Geometry check sheet. Reference: the model listing, model coordinates, mm. Face numbers are marked on the shaded views. A direction names the side the tool comes from. Coordinates: 2 decimals unless noted, no trailing zeros. Loops run counter-clockwise (first coordinate to the right, second up) from the corner with the lowest first, then second, coordinate; pieces in that order, holes last.
from build123d import *
from OCP.BRepFilletAPI import BRepFilletAPI_MakeChamfer

# Parameters (mm, degrees)
EXTRUDE_1_DEPTH                  = 11.1
CUT_EXTRUDE_1_DEPTH              = 7.7
SKETCH_13_R                      = 2.175
CUT_EXTRUDE_9_DEPTH              = 7.7
CUT_EXTRUDE_10_REACH             = 14.986
SKETCH_3_W                       = 1.5
SKETCH_3_H                       = 1.2
CUT_EXTRUDE_10_DIRECTION_2_REACH = 14.986
SKETCH_14_W                      = 1.5
SKETCH_14_H                      = 4
EXTRUDE_5_DEPTH                  = 1.2
EXTRUDE_START                    = 6.5
SKETCH_5_R                       = 2.175
EXTRUDE_3_DEPTH                  = 6.5
SKETCH_10_R                      = 2.15
CUT_EXTRUDE_7_DEPTH              = 6.5
SKETCH_16_R                      = 1.25
SKETCH_18_R                      = 1.25
EXTRUDE_7_DEPTH                  = 2
EXTRUDE_8_DEPTH                  = 8.1
EXTRUDE_START_2                  = -2.1
EXTRUDE_9_DEPTH                  = 2.1
SKETCH_21_W                      = 10.2
SKETCH_21_H                      = 2.025
EXTRUDE_12_DEPTH                 = 1
SKETCH_22_W                      = 0.6
SKETCH_22_H                      = 1.6
CUT_EXTRUDE_12_DEPTH             = 21.530769591
SKETCH_23_W                      = 0.7
SKETCH_23_H                      = 0.7
CUT_EXTRUDE_13_DEPTH             = 21.530769591
EXTRUDE_13_DEPTH                 = 2
EXTRUDE_13_DEPTH_BACK            = 7.6
SKETCH_24_W                      = 0.6
SKETCH_24_H                      = 1.6
EXTRUDE_14_DEPTH                 = 0.5
CHAMFER_2_SIZE                   = 1
CHAMFER_2_SIZE2                  = 0.577350269
CHAMFER_3_SIZE                   = 0.5
SKETCH_26_W                      = 9.9
SKETCH_26_H                      = 1.6
CUT_EXTRUDE_14_DEPTH             = 0.7
FILLET_4_R                       = 0.3
CUT_EXTRUDE_15_DEPTH             = 20.811738944
CUT_EXTRUDE_15_DEPTH_BACK        = 20.811738944
FILLET_5_R                       = 1


with BuildPart() as part:
    # Эскиз1 → Бобышка-Вытянуть1 (new body)
    with BuildSketch(Plane.XY):
        Polygon((-7.75, 1.221572875), (-7.75, -1.221572875), (-4.921572875, -4.05), (7.75, -4.05), (7.75, 4.05), (-4.921572875, 4.05), align=None)
    extrude(amount=EXTRUDE_1_DEPTH)

    # Эскиз2 → Вырез-Вытянуть1 (cut)
    with BuildSketch(Plane(origin=(0, 0, 0), x_dir=(-1, 0, 0), z_dir=(0, 0, -1))):
        Polygon((-7.75, 4.05), (-7.75, -4.05), (4.921572875, -4.05), (7.75, -1.221572875), (7.75, 1.221572875), (4.921572875, 4.05), align=None)
        Polygon((4.631623382, 3.35), (7.05, 0.931623382), (7.05, -0.931623382), (4.631623382, -3.35), (-7.05, -3.35), (-7.05, 3.35), align=None, mode=Mode.SUBTRACT)
    extrude(amount=-CUT_EXTRUDE_1_DEPTH, mode=Mode.SUBTRACT)

    # Эскиз13 → Вырез-Вытянуть9 (cut)
    with BuildSketch(Plane(origin=(0, 0, 0), x_dir=(-1, 0, 0), z_dir=(0, 0, -1))):
        with Locations((-3.6, 0)):
            Circle(SKETCH_13_R)
        with Locations((3.6, 0)):
            Circle(SKETCH_13_R)
    extrude(amount=-CUT_EXTRUDE_9_DEPTH, mode=Mode.SUBTRACT)

    # Вырез-Вытянуть10: up to this face of the body (flat: up to its plane)
    cut_extrude_10_end = Plane(part.part.faces().sort_by_distance((-3.6, 0, 7.7))[0])
    # Эскиз3 → Вырез-Вытянуть10 (cut, up to the picked face)
    with BuildSketch(Plane(origin=(0, 0, 1.5), x_dir=(-1, 0, 0), z_dir=(0, 0, -1)), mode=Mode.PRIVATE) as cut_extrude_10_sk1:
        with Locations((0, 2.75)):
            Rectangle(SKETCH_3_W, SKETCH_3_H)
    cut_extrude_10_tool1 = split(extrude(cut_extrude_10_sk1.sketch, amount=-CUT_EXTRUDE_10_REACH, mode=Mode.PRIVATE), bisect_by=cut_extrude_10_end, keep=Keep.BOTH, mode=Mode.PRIVATE)
    add(cut_extrude_10_tool1.solids().sort_by(Axis((0, 2.75, 1.5), (0, 0, 1)))[0], mode=Mode.SUBTRACT)

    # Вырез-Вытянуть10 direction 2: up to this face of the body (flat: up to its plane)
    cut_extrude_10_direction_2_end = Plane(part.part.faces().sort_by_distance((0.620013342, 0, 0))[0])
    # Эскиз3 → Вырез-Вытянуть10 direction 2 (cut, up to the picked face)
    with BuildSketch(Plane(origin=(0, 0, 1.5), x_dir=(-1, 0, 0), z_dir=(0, 0, -1)), mode=Mode.PRIVATE) as cut_extrude_10_direction_2_sk1:
        with Locations((0, 2.75)):
            Rectangle(SKETCH_3_W, SKETCH_3_H)
    cut_extrude_10_direction_2_tool1 = split(extrude(cut_extrude_10_direction_2_sk1.sketch, amount=CUT_EXTRUDE_10_DIRECTION_2_REACH, mode=Mode.PRIVATE), bisect_by=cut_extrude_10_direction_2_end, keep=Keep.BOTH, mode=Mode.PRIVATE)
    add(cut_extrude_10_direction_2_tool1.solids().sort_by(Axis((0, 2.75, 1.5), (0, 0, -1)))[0], mode=Mode.SUBTRACT)

    # Эскиз14 → Бобышка-Вытянуть5 (add)
    with BuildSketch(Plane(origin=(0, 0, 0), x_dir=(-1, 0, 0), z_dir=(0, 0, -1))):
        with Locations((0, 0.15)):
            Rectangle(SKETCH_14_W, SKETCH_14_H)
    extrude(amount=EXTRUDE_5_DEPTH)

    # Эскиз5 → Бобышка-Вытянуть3 (add)
    with BuildSketch(Plane(origin=(0, 0, 7.7), x_dir=(-1, 0, 0), z_dir=(0, 0, -1)).offset(EXTRUDE_START)):
        with Locations((3.6, 0)):
            Circle(SKETCH_5_R)
        with Locations((-3.6, 0)):
            Circle(SKETCH_5_R)
    extrude(amount=-EXTRUDE_3_DEPTH)

    # Эскиз10 → Вырез-Вытянуть7 (cut)
    with BuildSketch(Plane(origin=(0, 0, 1.2), x_dir=(-1, 0, 0), z_dir=(0, 0, -1))):
        with Locations((-3.6, 0)):
            Circle(SKETCH_10_R)
        with Locations((3.6, 0)):
            Circle(SKETCH_10_R)
    extrude(amount=-CUT_EXTRUDE_7_DEPTH, mode=Mode.SUBTRACT)

    # По траектории1: sweep along a path in Эскиз17
    with BuildLine(Plane(origin=(0, 0, 0), x_dir=(0, 0, -1), z_dir=(1, 0, 0))) as sweep_1_path:
        ThreePointArc((-15.15, 4.05), (-13.963782464, 1.186217536), (-11.1, 0))
    # Эскиз16 → По траектории1 (sweep)
    with BuildSketch(Plane.XY.offset(11.1)):
        with Locations((3.6, 0)):
            Circle(SKETCH_16_R)
        with Locations((-3.6, 0)):
            Circle(SKETCH_16_R)
    sweep(path=sweep_1_path.line)

    # Эскиз18 → Бобышка-Вытянуть7 (add)
    with BuildSketch(Plane(origin=(0, 4.05, 0), x_dir=(1, 0, 0), z_dir=(0, 1, 0))):
        with Locations(Location((3.6, -15.15, 0), (0, 0, 270))):
            Circle(SKETCH_18_R)
        with Locations(Location((-3.6, -15.15, 0), (0, 0, 270))):
            Circle(SKETCH_18_R)
    extrude(amount=EXTRUDE_7_DEPTH)

    # Эскиз19 → Бобышка-Вытянуть8 (add)
    with BuildSketch(Plane(origin=(0, 4.05, 0), x_dir=(1, 0, 0), z_dir=(0, 1, 0))):
        with BuildLine():
            ThreePointArc((5.25, -17.2), (7.100752265, -14.396209945), (7.75, -11.1))
            Line((7.75, -11.1), (5.1, -11.1))
            Line((5.1, -11.1), (5.1, -15.15))
            ThreePointArc((5.1, -15.15), (3.6, -16.65), (2.1, -15.15))
            Line((2.1, -15.15), (2.1, -11.1))
            Line((2.1, -11.1), (-2.1, -11.1))
            Line((-2.1, -11.1), (-2.1, -15.15))
            ThreePointArc((-2.1, -15.15), (-3.6, -16.65), (-5.1, -15.15))
            Line((-5.1, -15.15), (-5.1, -11.1))
            Line((-5.1, -11.1), (-4.921572875, -11.1))
            Line((-4.921572875, -11.1), (-4.921572875, -7.7))
            Line((-4.921572875, -7.7), (-7.75, -7.7))
            Line((-7.75, -7.7), (-7.75, -11.1))
            ThreePointArc((-7.75, -11.1), (-7.100752265, -14.396209945), (-5.25, -17.2))
            Line((-5.25, -17.2), (5.25, -17.2))
        make_face()
    extrude(amount=-EXTRUDE_8_DEPTH)

    # Эскиз20 → Бобышка-Вытянуть9 (add)
    with BuildSketch(Plane.XZ.offset(4.05).offset(EXTRUDE_START_2)):
        with BuildLine():
            Line((-7.75, 7.7), (7.75, 7.7))
            Line((7.75, 7.7), (7.75, 11.1))
            ThreePointArc((7.75, 11.1), (7.100752265, 14.396209945), (5.25, 17.2))
            Line((5.25, 17.2), (-5.25, 17.2))
            ThreePointArc((-5.25, 17.2), (-7.100752265, 14.396209945), (-7.75, 11.1))
            Line((-7.75, 11.1), (-7.75, 7.7))
        make_face()
    extrude(amount=EXTRUDE_9_DEPTH)

    # Эскиз21 → Бобышка-Вытянуть12 (add)
    with BuildSketch(Plane(origin=(0, 4.05, 0), x_dir=(1, 0, 0), z_dir=(0, 1, 0))):
        with Locations((0, -12.1125)):
            Rectangle(SKETCH_21_W, SKETCH_21_H)
    extrude(amount=-EXTRUDE_12_DEPTH)

    # Эскиз22 → Вырез-Вытянуть12 (cut, through all)
    with BuildSketch(Plane(origin=(0, 4.05, 0), x_dir=(1, 0, 0), z_dir=(0, 1, 0))):
        with Locations((-6.75, -9.15)):
            Rectangle(SKETCH_22_W, SKETCH_22_H)
        with Locations((6.75, -9.15)):
            Rectangle(SKETCH_22_W, SKETCH_22_H)
    extrude(amount=-CUT_EXTRUDE_12_DEPTH, mode=Mode.SUBTRACT)

    # Эскиз23 → Вырез-Вытянуть13 (cut, through all)
    with BuildSketch(Plane(origin=(0, 4.05, 0), x_dir=(1, 0, 0), z_dir=(0, 1, 0))):
        with Locations((-7.4, -9.15)):
            Rectangle(SKETCH_23_W, SKETCH_23_H)
        with Locations((7.4, -9.15)):
            Rectangle(SKETCH_23_W, SKETCH_23_H)
    extrude(amount=-CUT_EXTRUDE_13_DEPTH, mode=Mode.SUBTRACT)

    # Эскиз24 → Бобышка-Вытянуть13 (add, two sides: drawn at the far end of the back side and taken through both)
    with BuildSketch(Plane(origin=(0, 4.05, 0), x_dir=(1, 0, 0), z_dir=(0, 1, 0)).offset(-EXTRUDE_13_DEPTH_BACK)):
        with Locations((-6.75, -9.15)):
            Rectangle(SKETCH_24_W, SKETCH_24_H)
        with Locations((6.75, -9.15)):
            Rectangle(SKETCH_24_W, SKETCH_24_H)
    extrude(amount=EXTRUDE_13_DEPTH + EXTRUDE_13_DEPTH_BACK)

    # Эскиз25 → Бобышка-Вытянуть14 (add)
    with BuildSketch(Plane(origin=(0, 4.05, 0), x_dir=(1, 0, 0), z_dir=(0, 1, 0))):
        Polygon((-6.15, -8.05), (-7.35, -8.05), (-7.35, -8.8), (-7.05, -8.8), (-7.05, -8.35), (-6.45, -8.35), (-6.45, -9.95), (-7.05, -9.95), (-7.05, -9.5), (-7.35, -9.5), (-7.35, -10.25), (-6.15, -10.25), align=None)
        Polygon((7.35, -8.05), (6.15, -8.05), (6.15, -10.25), (7.35, -10.25), (7.35, -9.5), (7.05, -9.5), (7.05, -9.95), (6.45, -9.95), (6.45, -8.35), (7.05, -8.35), (7.05, -8.8), (7.35, -8.8), align=None)
    extrude(amount=EXTRUDE_14_DEPTH)

    # Фаска2: one chamfer whose edges measure the first distance from different faces: ONE call of the kernel's chamfer builder (chamfer() names one face for all edges)
    chamfer_2_edges_1 = [part.edges().sort_by_distance(p)[0] for p in [
        (-6.75, 6.05, 9.95),
    ]]
    chamfer_2_side_1 = [part.faces().sort_by_distance(p)[0] for p in [
        (-6.75, 5.3, 9.95),
    ]]
    chamfer_2_edges_2 = [part.edges().sort_by_distance(p)[0] for p in [
        (-6.75, 6.05, 8.35),
    ]]
    chamfer_2_side_2 = [part.faces().sort_by_distance(p)[0] for p in [
        (-6.75, 5.3, 8.35),
    ]]
    chamfer_2_edges_3 = [part.edges().sort_by_distance(p)[0] for p in [
        (6.75, 6.05, 9.95),
    ]]
    chamfer_2_side_3 = [part.faces().sort_by_distance(p)[0] for p in [
        (6.75, 5.3, 9.95),
    ]]
    chamfer_2_edges_4 = [part.edges().sort_by_distance(p)[0] for p in [
        (6.75, 6.05, 8.35),
    ]]
    chamfer_2_side_4 = [part.faces().sort_by_distance(p)[0] for p in [
        (6.75, 5.3, 8.35),
    ]]
    chamfer_2 = BRepFilletAPI_MakeChamfer(part.part.solid().wrapped)
    for e in chamfer_2_edges_1:
        chamfer_2.Add(CHAMFER_2_SIZE, CHAMFER_2_SIZE2, e.wrapped, chamfer_2_side_1[0].wrapped)  # the first distance lies on this face
    for e in chamfer_2_edges_2:
        chamfer_2.Add(CHAMFER_2_SIZE, CHAMFER_2_SIZE2, e.wrapped, chamfer_2_side_2[0].wrapped)  # the first distance lies on this face
    for e in chamfer_2_edges_3:
        chamfer_2.Add(CHAMFER_2_SIZE, CHAMFER_2_SIZE2, e.wrapped, chamfer_2_side_3[0].wrapped)  # the first distance lies on this face
    for e in chamfer_2_edges_4:
        chamfer_2.Add(CHAMFER_2_SIZE, CHAMFER_2_SIZE2, e.wrapped, chamfer_2_side_4[0].wrapped)  # the first distance lies on this face
    add(Compound.cast(chamfer_2.Shape()), mode=Mode.REPLACE)

    # Фаска3
    chamfer_3_edges = [part.edges().sort_by_distance(p)[0] for p in [
        (3.6, 6.05, 13.9),
        (-3.6, 6.05, 13.9),
    ]]
    chamfer(chamfer_3_edges, length=CHAMFER_3_SIZE)

    # Эскиз26 → Вырез-Вытянуть14 (cut)
    with BuildSketch(Plane.XZ.offset(4.05)):
        with Locations((0, 9.15)):
            Rectangle(SKETCH_26_W, SKETCH_26_H)
    extrude(amount=-CUT_EXTRUDE_14_DEPTH, mode=Mode.SUBTRACT)

    # Скругление4
    fillet_4_edges = [part.edges().sort_by_distance(p)[0] for p in [
        (7.75, -4.05, 8.25),
        (-7.75, -4.05, 8.25),
        (7.05, 3.35, 3.85),
        (7.05, -3.35, 3.85),
        (-4.631623382, -3.35, 3.85),
        (-7.05, -0.931623382, 3.85),
        (-7.05, 0.931623382, 3.85),
        (-4.631623382, 3.35, 3.85),
        (4.95, -3.7, 9.95),
        (4.95, -3.7, 8.35),
        (-4.95, -3.7, 8.35),
        (-4.95, -3.7, 9.95),
    ]]
    fillet(fillet_4_edges, radius=FILLET_4_R)

    # Эскиз27 → Вырез-Вытянуть15 (cut, two sides: drawn at the far end of the back side and taken through both)
    with BuildSketch(Plane(origin=(0, 0, 0), x_dir=(0, 0, -1), z_dir=(1, 0, 0)).offset(-CUT_EXTRUDE_15_DEPTH_BACK)):
        with BuildLine():
            Line((-11.1, -4.05), (-17.2, -4.05))
            Line((-17.2, -4.05), (-17.2, -1.55))
            ThreePointArc((-17.2, -1.55), (-14.396209945, -3.400752265), (-11.1, -4.05))
        make_face()
    extrude(amount=CUT_EXTRUDE_15_DEPTH + CUT_EXTRUDE_15_DEPTH_BACK, mode=Mode.SUBTRACT)

    # Скругление5
    fillet_5_edges = [part.edges().sort_by_distance(p)[0] for p in [
        (7.75, -4.05, 10.3),
        (-7.75, -4.05, 10.3),
        (5.25, 1.25, 17.2),
        (-5.25, 1.25, 17.2),
        (7.027776856, -3.327776856, 14.568936562),
        (-7.027776856, -3.327776856, 14.568936562),
        (0, -1.55, 17.2),
    ]]
    fillet(fillet_5_edges, radius=FILLET_5_R)


solid = part.part
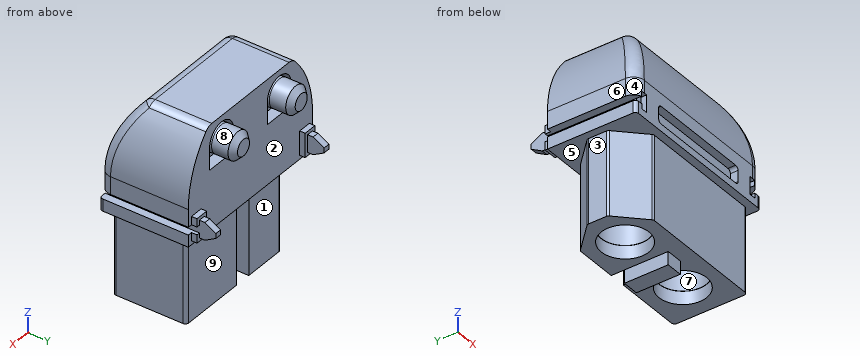
1) Depth check by flat-ended pin: pin 1 (0.9 mm diameter, centred on x = 3.5, z = 12.5, fed in from +Y); pin 2 (2 mm diameter, centred on y = 1, z = 7, fed in from +X); pin 3 (6 mm diameter, centred on x = 0, z = 14, fed in from +Y); pin 4 (0.6 mm diameter, centred on y = 0.5, z = -0.5, fed in from +X). Enter the tip coordinate at first touch or a pass-through.
Data:
pin 1: stops at y = 4.05
pin 2: stops at x = 7.75
pin 3: stops at y = 6.02
pin 4: stops at x = 0.75
2) Section check A-A on z = 4.5. Record the cut outline in (x, y), and give its area (3 significant figures).
Data:
outline: (-7.05, -0.81) arc R0.3 ccw to (-6.96, -1.02) - (-4.72, -3.26) arc R0.3 ccw to (-4.51, -3.35) - (6.75, -3.35) arc R0.3 ccw to (7.05, -3.05) - (7.05, 3.05) arc R0.3 ccw to (6.75, 3.35) - (0.75, 3.35) - (0.75, 2.15) - (-0.75, 2.15) - (-0.75, 3.35) - (-4.51, 3.35) arc R0.3 ccw to (-4.72, 3.26) - (-6.96, 1.02) arc R0.3 ccw to (-7.05, 0.81) - close; hole circle Ø4.3 at (-3.6, 0); hole circle Ø4.3 at (3.6, 0)
area: 57.7 mm2
3) Access from +Z, -Z, +X, -X, +Y, -Y to the whole of each face (thin tool, end or side, straight path). Record for the marked faces 1, 2, 3, 4 and 5.
Data:
face 1: -Z, +X, -X, +Y
face 2: +Y
face 3: -Z, -X, +Y, -Y
face 4: +Z, -X, -Y
face 5: -Z
4) Material ranges on probe 1 along X at (y, z) = (0, 4); probe 2 along Y at (x, z) = (3.6, 0.3) (3 decimals); probe 3 along X at (y, z) = (-1.25, 13.5), recorded low to high.
Data:
probe 1: x = -7.05 to -5.75, -1.45 to 1.45, 5.75 to 7.05
probe 2: y = -3.35 to -2.175, 2.175 to 3.35
probe 3: x = -7.41 to -5.1, -2.1 to 2.1, 5.1 to 7.41
5) Mould release check, pull along X, two halves, no side actions. Record for the marked faces 6, 7, 8 and 9: +X half, -X half, draft (parallel to the pull), parting line (faces both ways), or undercut.
Data:
face 6: -X half
face 7: undercut
face 8: undercut
face 9: draft
6) Section check B-B on y = 0. Count the separate pieces of the cut face and the enclosed holes in it, and give its area (3 significant figures).
Data:
separate pieces: 1
enclosed holes: 2
area: 164 mm2
